Check sheet for the modelled part. Datum: model origin and axes. Units: mm. Round coordinates to 2 decimals unless told otherwise and drop trailing zeros. Write each loop counter-clockwise with the first axis right and the second up, starting at its lowest first coordinate (ties: lowest second). Pieces come first, ordered by that corner, then holes.
Item 1: Material ranges on line 1 (Y direction, x = -17, z = -1); line 2 (X direction, y = 59, z = 0.5); line 3 (X direction, y = 43, z = 2.5), recorded low to high.
Item 2: Cross-section at C-C on x = 68. Enter the section's corners in (y, z) (3 decimals).
Item 3: Cross-section at B-B on y = 71.5. Enter the section's corners in (x, z) (3 decimals).
Item 4: Go/stop test with flat-tipped pins: pin 1 Ø2.5 at (x, y) = (68, 102) entering from +Z; pin 2 Ø1.9 at (y, z) = (71.5, 0) entering from +X. Record where each tip stops, or that it passes through.
Item 5: Cross-section at A-A on y = 116. Enter the section's corners in (x, z) (3 decimals), plus the area to 3 significant figures.
Item 6: Cross-section at D-D on z = -0.75. Count the separate pieces of the cut face and the enclosed holes in it, plus the area to 3 significant figures.
from build123d import *

# Parameters (mm, degrees)
BOSS_EXTRUDE1_DEPTH     = 3.175
CUT_EXTRUDE2_DEPTH      = 150.86267881
CUT_EXTRUDE2_DEPTH_BACK = 150.86267881
SKETCH3_R               = 1.25
CUT_EXTRUDE6_DEPTH      = 150.86267881
CUT_EXTRUDE6_DEPTH_BACK = 150.86267881
SKETCH12_R              = 2.25
CUT_EXTRUDE7_DEPTH      = 150.86267881
CUT_EXTRUDE7_DEPTH_BACK = 150.86267881
FILLET4_R               = 4


with BuildPart() as part:
    # Sketch1 → Boss-Extrude1 (new, symmetric)
    with BuildSketch(Plane.XY):
        with BuildLine():
            Line((87.5, 121.5), (-87.5, 121.5))
            Line((-87.5, 121.5), (-87.5, 96.5))
            Line((-87.5, 96.5), (-43.327910637, -16.880229852))
            ThreePointArc((-43.327910637, -16.880229852), (0, -46.5), (43.327910637, -16.880229852))
            Line((43.327910637, -16.880229852), (87.5, 96.5))
            Line((87.5, 96.5), (87.5, 121.5))
        make_face()
    extrude(amount=BOSS_EXTRUDE1_DEPTH, both=True)

    # Sketch3 → Cut-Extrude2 (cut, two sides: drawn at the far end of the back side and taken through both)
    with BuildSketch(Plane(origin=(0, 0, -3.175), x_dir=(-1, 0, 0), z_dir=(0, 0, -1)).offset(-CUT_EXTRUDE2_DEPTH_BACK)):
        with Locations((17.440159599, -16.121517706)):
            Circle(SKETCH3_R)
        with Locations((22.282044228, -8.220280106)):
            Circle(SKETCH3_R)
        with Locations((9.943168767, -21.568400378)):
            Circle(SKETCH3_R)
        with Locations((0.932420624, -23.731689611)):
            Circle(SKETCH3_R)
        with Locations((-8.220280106, -22.282044228)):
            Circle(SKETCH3_R)
        with Locations((-16.121517706, -17.440159599)):
            Circle(SKETCH3_R)
        with Locations((-21.568400378, -9.943168767)):
            Circle(SKETCH3_R)
        with Locations((-23.731689611, -0.932420624)):
            Circle(SKETCH3_R)
        with Locations((-22.282044228, 8.220280106)):
            Circle(SKETCH3_R)
        with Locations((-17.440159599, 16.121517706)):
            Circle(SKETCH3_R)
        with Locations((-9.943168767, 21.568400378)):
            Circle(SKETCH3_R)
        with Locations((-0.932420624, 23.731689611)):
            Circle(SKETCH3_R)
        with Locations((8.220280106, 22.282044228)):
            Circle(SKETCH3_R)
        with Locations((16.121517706, 17.440159599)):
            Circle(SKETCH3_R)
        with Locations((21.568400378, 9.943168767)):
            Circle(SKETCH3_R)
        with Locations((23.731689611, 0.932420624)):
            Circle(SKETCH3_R)
    extrude(amount=CUT_EXTRUDE2_DEPTH + CUT_EXTRUDE2_DEPTH_BACK, mode=Mode.SUBTRACT)

    # Sketch12 → Cut-Extrude6 (cut, two sides: drawn at the far end of the back side and taken through both)
    with BuildSketch(Plane(origin=(0, 0, -3.175), x_dir=(-1, 0, 0), z_dir=(0, 0, -1)).offset(-CUT_EXTRUDE6_DEPTH_BACK)):
        with Locations((-7, 102)):
            Circle(SKETCH12_R)
        with Locations((7, 102)):
            Circle(SKETCH12_R)
        with Locations((7, 116)):
            Circle(SKETCH12_R)
        with Locations((-82, 116)):
            Circle(SKETCH12_R)
        with Locations((-68, 116)):
            Circle(SKETCH12_R)
        with Locations((-68, 102)):
            Circle(SKETCH12_R)
        with Locations((-82, 102)):
            Circle(SKETCH12_R)
        with Locations(Location((82, 102, 0), (0, 0, 180))):
            Circle(SKETCH12_R)
        with Locations(Location((68, 102, 0), (0, 0, 180))):
            Circle(SKETCH12_R)
        with Locations(Location((68, 116, 0), (0, 0, 180))):
            Circle(SKETCH12_R)
        with Locations(Location((82, 116, 0), (0, 0, 180))):
            Circle(SKETCH12_R)
        with Locations((-7, 116)):
            Circle(SKETCH12_R)
    extrude(amount=CUT_EXTRUDE6_DEPTH + CUT_EXTRUDE6_DEPTH_BACK, mode=Mode.SUBTRACT)

    # Sketch13 → Cut-Extrude7 (cut, two sides: drawn at the far end of the back side and taken through both)
    with BuildSketch(Plane(origin=(0, 0, -3.175), x_dir=(-1, 0, 0), z_dir=(0, 0, -1)).offset(-CUT_EXTRUDE7_DEPTH_BACK)):
        with BuildLine():
            Line((-39.473357495, 24.578528192), (-64.591776998, 89.0520955))
            ThreePointArc((-64.591776998, 89.0520955), (-57.549704921, 94.796577819), (-53.354481954, 102.85821292))
            Line((-53.354481954, 102.85821292), (-21.645518046, 102.85821292))
            ThreePointArc((-21.645518046, 102.85821292), (-17.06210253, 94.332530646), (-9.32089354, 88.521451623))
            Line((-9.32089354, 88.521451623), (-9.32089354, 45.556239349))
            ThreePointArc((-9.32089354, 45.556239349), (-26.556276563, 38.170855048), (-39.473357495, 24.578528192))
        make_face()
        with BuildLine():
            Line((39.473357495, 24.578528192), (64.555315361, 88.958506339))
            ThreePointArc((64.555315361, 88.958506339), (57.499891336, 94.745342648), (53.322832732, 102.85821292))
            Line((53.322832732, 102.85821292), (21.645518046, 102.85821292))
            ThreePointArc((21.645518046, 102.85821292), (17.06210253, 94.332530646), (9.32089354, 88.521451623))
            Line((9.32089354, 88.521451623), (9.32089354, 45.556239349))
            ThreePointArc((9.32089354, 45.556239349), (26.556276563, 38.170855048), (39.473357495, 24.578528192))
        make_face()
    extrude(amount=CUT_EXTRUDE7_DEPTH + CUT_EXTRUDE7_DEPTH_BACK, mode=Mode.SUBTRACT)

    # Fillet4
    fillet4_edges = [part.edges().sort_by_distance(p)[0] for p in [
        (-53.322832732, 102.85821292, 0),
        (-64.555315361, 88.958506339, 0),
        (-39.473357495, 24.578528192, 0),
        (-9.32089354, 45.556239349, 0),
        (-9.32089354, 88.521451623, 0),
        (-21.645518046, 102.85821292, 0),
        (64.591776998, 89.0520955, 0),
        (53.354481954, 102.85821292, 0),
        (21.645518046, 102.85821292, 0),
        (9.32089354, 88.521451623, 0),
        (9.32089354, 45.556239349, 0),
        (39.473357495, 24.578528192, 0),
    ]]
    fillet(fillet4_edges, radius=FILLET4_R)


solid = part.part
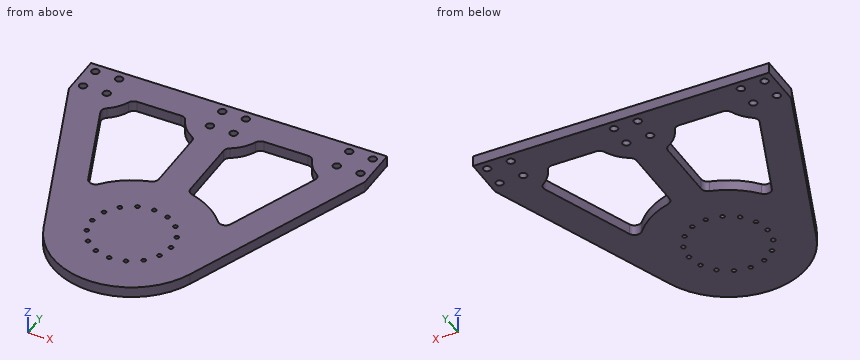
Response values:
1. line 1: y = -43.28 to -17.29, -14.95 to 16.55, 18.33 to 43.28, 94.26 to 121.5
1. line 2: x = -72.89 to -52.88, -9.32 to 9.32, 52.88 to 72.89
1. line 3: x = -66.66 to -46.65, -17.7 to 17.7, 46.65 to 66.66
2. outline: (46.448, -3.175) - (99.75, -3.175) - (99.75, 3.175) - (46.448, 3.175) - close; (104.25, -3.175) - (113.75, -3.175) - (113.75, 3.175) - (104.25, 3.175) - close; (118.25, -3.175) - (121.5, -3.175) - (121.5, 3.175) - (118.25, 3.175) - close
3. outline: (-77.76, -3.175) - (-57.754, -3.175) - (-57.754, 3.175) - (-77.76, 3.175) - close; (-9.321, -3.175) - (9.321, -3.175) - (9.321, 3.175) - (-9.321, 3.175) - close; (57.754, -3.175) - (77.76, -3.175) - (77.76, 3.175) - (57.754, 3.175) - close
4. pin 1: passes through
4. pin 2: stops at x = 78.13
5. outline: (-87.5, -3.175) - (-84.25, -3.175) - (-84.25, 3.175) - (-87.5, 3.175) - close; (-79.75, -3.175) - (-70.25, -3.175) - (-70.25, 3.175) - (-79.75, 3.175) - close; (-65.75, -3.175) - (-9.25, -3.175) - (-9.25, 3.175) - (-65.75, 3.175) - close; (-4.75, -3.175) - (4.75, -3.175) - (4.75, 3.175) - (-4.75, 3.175) - close; (9.25, -3.175) - (65.75, -3.175) - (65.75, 3.175) - (9.25, 3.175) - close; (70.25, -3.175) - (79.75, -3.175) - (79.75, 3.175) - (70.25, 3.175) - close; (84.25, -3.175) - (87.5, -3.175) - (87.5, 3.175) - (84.25, 3.175) - close
5. area: 940 mm2
6. separate pieces: 1
6. enclosed holes: 30
6. area: 15,100 mm2
